Build history of the part. All positions in model axes, mm. Round coordinates to 2 decimals unless told otherwise and drop trailing zeros. Write each loop counter-clockwise with the first axis right and the second up, starting at its lowest first coordinate (ties: lowest second). Pieces come first, ordered by that corner, then holes.
1) Saw through at D-D (y = 0). Write the cut outline in (x, z), plus the area to 3 significant figures.
2) Flat gauge pin, fed straight in: pin 1 (0.6 mm diameter, centred on x = 0, z = -0.5, fed in from -Y). Where does the tip first touch, or does it go through?
3) Saw through at A-A (z = -0.5). Write the cut outline in (x, y), plus the area to 3 significant figures.
4) Saw through at B-B (x = 1.35). Write the cut outline in (y, z).
5) Saw through at C-C (z = 5). Write the cut outline in (x, y), plus the area to 3 significant figures.
6) Wall check: probe 1 along Y at (x, z) = (2.5, 1.75); probe 2 along Z at (x, y) = (1.85, -1.2); probe 3 along Z at (x, y) = (3.25, 0.95). Give the ranges that are in metal, low to high.
from build123d import *

# Parameters (mm, degrees)
PAD001_DEPTH = 0.2
PAD_DEPTH    = 6.9
FILLET_R     = 2


with BuildPart() as pad001:
    # Sketch002 → Pad001 (new body, symmetric)
    with BuildSketch(Plane.XZ):
        Polygon((-0.25, 3), (0.25, 3), (0.25, 2), (0.4, 2), (0.4, 0.5), (0.25, 0.5), (0.25, -3), (-0.25, -3), (-0.25, 0.5), (-0.4, 0.5), (-0.4, 2), (-0.25, 2), align=None)
        Polygon((2.29, 3), (2.79, 3), (2.79, 2), (2.94, 2), (2.94, 0.5), (2.79, 0.5), (2.79, -3), (2.29, -3), (2.29, 0.5), (2.14, 0.5), (2.14, 2), (2.29, 2), align=None)
    extrude(amount=PAD001_DEPTH, both=True)


with BuildPart() as obj1:
    # Sketch → Pad (new body)
    with BuildSketch(Plane.XY.offset(3)):
        with BuildLine():
            Line((-0.754846, -1.35), (3.294846, -1.35))
            ThreePointArc((3.294846, -1.35), (3.82, 0.2), (3.294846, 1.75))
            Line((3.294846, 1.75), (-0.754846, 1.75))
            ThreePointArc((-0.754846, 1.75), (-1.28, 0.2), (-0.754846, -1.35))
        make_face()
    extrude(amount=PAD_DEPTH)

    # Fillet
    fillet_edges = [obj1.edges().sort_by_distance(p)[0] for p in [
        (1.27, 1.75, 9.9),
    ]]
    fillet(fillet_edges, radius=FILLET_R)

    add(pad001.part)


solid = obj1.part
Evaluation:
1. outline: (-1.27, 3) - (-0.25, 3) - (-0.25, 2) - (-0.4, 2) - (-0.4, 0.5) - (-0.25, 0.5) - (-0.25, -3) - (0.25, -3) - (0.25, 0.5) - (0.4, 0.5) - (0.4, 2) - (0.25, 2) - (0.25, 3) - (2.29, 3) - (2.29, 2) - (2.14, 2) - (2.14, 0.5) - (2.29, 0.5) - (2.29, -3) - (2.79, -3) - (2.79, 0.5) - (2.94, 0.5) - (2.94, 2) - (2.79, 2) - (2.79, 3) - (3.81, 3) - (3.81, 9.88) - (-1.27, 9.88) - close
1. area: 41.9 mm2
2. pin 1: stops at y = -0.2
3. outline: (-0.25, -0.2) - (0.25, -0.2) - (0.25, 0.2) - (-0.25, 0.2) - close; (2.29, -0.2) - (2.79, -0.2) - (2.79, 0.2) - (2.29, 0.2) - close
3. area: 0.400 mm2
4. outline: (-1.35, 3) - (1.75, 3) - (1.75, 7.9) arc R2 ccw to (-0.25, 9.9) - (-1.35, 9.9) - close
5. outline: (-0.75, -1.35) - (3.29, -1.35) arc R2.55 ccw to (3.29, 1.75) - (-0.75, 1.75) arc R2.55 ccw to start
5. area: 14.8 mm2
6. probe 1: y = -0.2 to 0.2
6. probe 2: z = 3 to 9.9
6. probe 3: z = 3 to 9.5
